Input: part model. Units: mm. Frame: model coordinates. Face numbers are marked on the shaded views. A direction names the side the tool comes from. Coordinates: 2 decimals unless noted, no trailing zeros. Write each loop counter-clockwise with the first axis right and the second up, starting at its lowest first coordinate (ties: lowest second). Pieces come first, ordered by that corner, then holes. Notation, with made-up numbers: M -32,-11.5 L 3,-11.5 A14 cw 3,-7.5 Z; hole C 83.25,63.25 d8. An arc over 180 degrees is marked long. Use one line per item in the form item = value.
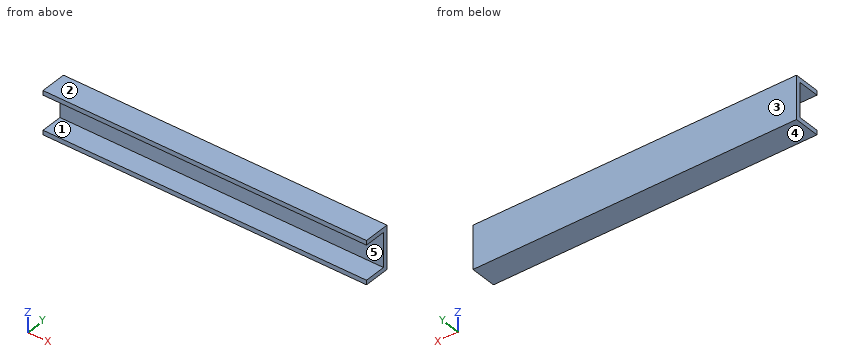
from build123d import *

# Parameters (mm, degrees)
F0_W     = 571.5
F0_H     = 76.2
F1_DEPTH = 7.9375
F2_W     = 571.5
F2_H     = 7.9375
F3_DEPTH = 38.1


with BuildPart() as f1:
    # F0 (on Front) → F1 (new body)
    with BuildSketch(Plane.XZ):
        with Locations((285.75, 38.1)):
            Rectangle(F0_W, F0_H)
    extrude(amount=-F1_DEPTH)

    # F2 (on Front) → F3 (join)
    with BuildSketch(Plane.XZ):
        with Locations((285.75, 72.23125)):
            Rectangle(F2_W, F2_H)
        with Locations((285.75, 3.96875)):
            Rectangle(F2_W, F2_H)
    extrude(amount=F3_DEPTH)


solid = f1.part
(1) First-contact query: pin 1 Ø6 at (x, z) = (148.5, 29.5) entering from -Y; pin 2 Ø5 at (x, y) = (118, -7) entering from -Z. Flat tips, straight axial feed; report the tip coordinate or a pass-through.
Computed:
pin_1 = 0
pin_2 = 0
(2) Pull-direction query (Z, two-part tool) for the marked faces 1, 2 and 3; classes: pulls with the +Z half, pulls with the -Z half, needs draft (parallel to the pull), parting line crosses it, or undercut.
Computed:
face_1 = undercut
face_2 = pulls with the +Z half
face_3 = needs draft
(3) Line query: probe 1 along Z at (x, y) = (467.5, -13); probe 2 along Y at (x, z) = (284.5, 10.5). Output: solid intervals per line, ascending.
Computed:
probe_1 = 0 to 7.94, 68.26 to 76.2
probe_2 = 0 to 7.94
(4) Set-up query: the marked faces 4 and 5. Return all of +Z, -Z, +X, -X, +Y, -Y with unobstructed straight access to the full face (end or side cutting, diameter ignored); none if empty.
Computed:
face_4 = -Z, +X, -X, +Y, -Y
face_5 = +X, -X, -Y
(5) Section query B-B on x = 363. Return the cut outline in (y, z), plus the area to 3 significant figures.
Computed:
outline = M -38.1,0 L 7.94,0 L 7.94,76.2 L -38.1,76.2 L -38.1,68.26 L 0,68.26 L 0,7.94 L -38.1,7.94 Z
area = 1,210 mm^2
(6) Section query C-C on z = 28. Return the cut outline in (x, y), plus the area to 3 significant figures.
Computed:
outline = M 0,0 L 571.5,0 L 571.5,7.94 L 0,7.94 Z
area = 4,540 mm^2
(7) Section query A-A on y = -29. Return the cut outline in (x, z).
Computed:
outline = M 0,0 L 571.5,0 L 571.5,7.94 L 0,7.94 Z; M 0,68.26 L 571.5,68.26 L 571.5,76.2 L 0,76.2 Z
